```python
from build123d import *

# Parameters (mm, degrees)
F2_SIZE2 = 0.2
F2_SIZE  = 10


with BuildPart() as f1:
    # F0 (on Front) → F1 (revolve)
    with BuildSketch(Plane.XZ):
        with BuildLine():
            Line((0, 44.181132), (0, 49.181134))
            Line((0, 49.181134), (-17, 49.181134))
            Line((-17, 49.181134), (-17, 79.181135))
            Line((-17, 79.181135), (-25, 79.181135))
            Line((-25, 79.181135), (-25, 39.181132))
            Line((-25, 39.181132), (-22, 39.181132))
            Line((-22, 39.181132), (-22, 29.181132))
            Line((-22, 29.181132), (-4.5, 29.181132))
            ThreePointArc((-4.5, 29.181132), (-3.792893, 28.888239), (-3.5, 28.181132))
            Line((-3.5, 28.181132), (-3.5, -30.818868))
            Line((-3.5, -30.818868), (-3.25, -30.818868))
            Line((-3.25, -30.818868), (-3.25, 44.181132))
            Line((-3.25, 44.181132), (0, 44.181132))
        make_face()
    revolve(axis=Axis((0, 0, 1.49861), (0, 0, -1)))

    # F2
    f2_edges = [f1.edges().sort_by_distance(p)[0] for p in [
        (3.5, 0, -30.818868),
    ]]
    chamfer(f2_edges, length=F2_SIZE, length2=F2_SIZE2)


solid = f1.part
```
Source: CAD feature listing. Evaluate the final solid. Frame: model axes, mm. A direction names the side the tool comes from. Coordinates: 2 decimals unless noted, no trailing zeros. Loops run counter-clockwise (first coordinate to the right, second up) from the corner with the lowest first, then second, coordinate; pieces in that order, holes last. Notation, with made-up numbers: M -14,-3 L 28,-3 A14 ccw 28,1 Z; hole C 23,20 d6. An arc over 180 degrees is marked long. Use a Markdown table: item, result. Add a question column.
Q1. Draft query along Y for faces 3 (the flat face through (-1.7, -22.1, 39.181)), 4 (the cylindrical face through (-3.233, -1.341, 3.338)), 5 (the cylindrical face through (-9.139, 14.334, 64.391)), 6 (the flat face through (0, 0, 49.181)). Return one class per face: pulls with the +Y half, pulls with the -Y half, needs draft (parallel to the pull), parting line crosses it, or undercut.
Q2. Section query D-D, the plane y = 10.5. Return loops of the section in (x, z), and give its area (3 significant figures).
Q3. Section query C-C, the plane x = -8.5. Return loops of the section in (y, z), and give its area (3 significant figures).
Q4. Material intervals for L1, parallel to Y at x = 0, z = -13; L2, parallel to Y at x = 0, z = 58; L3, parallel to Z at x = -19.5, y = 1.5, sorted ascending.
Q5. Access query for faces 1 (the cylindrical face through (2.579, -1.978, 7.206)), 2 (the flat face through (-5.9, -16.3, 79.181)). Directions: +Z, -Z, +X, -X, +Y, -Y. A direction counts if a zero-diameter tool reaches every point of the face in a straight line with its end or side. Return the directions, or none.
Q6. Section query A-A, the plane z = 65.5. Return loops of the section in (x, y).
Q7. Section query B-B, the plane y = -19.5. Return loops of the section in (x, z), and give its area (3 significant figures).
Q8. First-contact query: pin 1 (6 mm diameter, centred on x = -3, y = 10, fed in from -Z); pin 2 (10 mm diameter, centred on x = 16.5, z = 40, fed in from -Y); pin 3 (5 mm diameter, centred on x = -0.5, y = 0, fed in from -Z); pin 4 (20.5 mm diameter, centred on x = 0, y = 0, fed in from -Z). Flat tips, straight axial feed; report the tip coordinate or a pass-through.
Result:
| question | item | result |
|---|---|---|
| 1 | face 3 | needs draft |
| 1 | face 4 | parting line crosses it |
| 1 | face 5 | undercut |
| 1 | face 6 | undercut |
| 2 | outline | M -22.69,39.18 L -19.33,39.18 L -19.33,29.18 L 19.33,29.18 L 19.33,39.18 L 22.69,39.18 L 22.69,79.18 L 13.37,79.18 L 13.37,49.18 L -13.37,49.18 L -13.37,79.18 L -22.69,79.18 Z |
| 2 | area | 1,400 mm2 |
| 3 | outline | M -23.51,39.18 L -20.29,39.18 L -20.29,29.18 L 20.29,29.18 L 20.29,39.18 L 23.51,39.18 L 23.51,79.18 L 14.72,79.18 L 14.72,49.18 L -14.72,49.18 L -14.72,79.18 L -23.51,79.18 Z |
| 3 | area | 1,400 mm2 |
| 4 | L1 | y = -3.5 to -3.25, 3.25 to 3.5 |
| 4 | L2 | y = -25 to -17, 17 to 25 |
| 4 | L3 | z = 29.18 to 79.18 |
| 5 | face 1 | -Z |
| 5 | face 2 | +Z, +X, -X, +Y, -Y |
| 6 | outline | C 0,0 d50; hole C 0,0 d34 |
| 7 | outline | M -15.64,39.18 L -10.19,39.18 L -10.19,29.18 L 10.19,29.18 L 10.19,39.18 L 15.64,39.18 L 15.64,79.18 L -15.64,79.18 Z |
| 7 | area | 1,460 mm2 |
| 8 | pin 1 | stops at z = 29.18 |
| 8 | pin 2 | stops at y = -22.2 |
| 8 | pin 3 | stops at z = 44.18 |
| 8 | pin 4 | stops at z = -30.82 |
